```python
from build123d import *

# Parameters (mm, degrees)
SKETCH_1_W          = 56
SKETCH_1_H          = 104
SKETCH_1_R          = 1.6
EXTRUDE_1_DEPTH     = 2
FILLET_1_R          = 3
CUT_EXTRUDE_1_DEPTH = 10
FILLET_2_R          = 2


with BuildPart() as part:
    # 草图1 → 凸台-拉伸1 (new body)
    with BuildSketch(Plane.XY):
        Rectangle(SKETCH_1_W, SKETCH_1_H)
        with Locations((-24, 48)):
            Circle(SKETCH_1_R, mode=Mode.SUBTRACT)
        with Locations((-24, -48)):
            Circle(SKETCH_1_R, mode=Mode.SUBTRACT)
        with Locations(Location((24, -48, 0), (0, 0, 180))):
            Circle(SKETCH_1_R, mode=Mode.SUBTRACT)
        with Locations(Location((24, 48, 0), (0, 0, 180))):
            Circle(SKETCH_1_R, mode=Mode.SUBTRACT)
    extrude(amount=EXTRUDE_1_DEPTH)

    # 圆角1
    fillet_1_edges = [part.edges().sort_by_distance(p)[0] for p in [
        (28, -52, 1),
        (-28, -52, 1),
        (-28, 52, 1),
        (28, 52, 1),
    ]]
    fillet(fillet_1_edges, radius=FILLET_1_R)

    # 草图2 → 切除-拉伸1 (cut)
    with BuildSketch(Plane.XY.offset(2)):
        Polygon((-20, 34.939835194), (-20, -34.939835194), (-3.324169566, 0), align=None)
        Polygon((-17.198557706, -43), (17.198557706, -43), (0, -6.96492671), align=None)
        Polygon((0, 6.96492671), (-17.198557706, 43), (17.198557706, 43), align=None)
        Polygon((3.324169566, 0), (20, 34.939835194), (20, -34.939835194), align=None)
    extrude(amount=-CUT_EXTRUDE_1_DEPTH, mode=Mode.SUBTRACT)

    # 圆角2
    fillet_2_edges = [part.edges().sort_by_distance(p)[0] for p in [
        (-3.324169566, 0, 1),
        (-20, -34.939835194, 1),
        (-20, 34.939835194, 1),
        (-17.198557706, -43, 1),
        (0, -6.96492671, 1),
        (17.198557706, -43, 1),
        (17.198557706, 43, 1),
        (0, 6.96492671, 1),
        (-17.198557706, 43, 1),
        (20, -34.939835194, 1),
        (3.324169566, 0, 1),
        (20, 34.939835194, 1),
    ]]
    fillet(fillet_2_edges, radius=FILLET_2_R)


solid = part.part
```
Input: part model. Units: mm. Frame: model coordinates. A direction names the side the tool comes from. Round coordinates to 2 decimals unless told otherwise and drop trailing zeros. Loops run counter-clockwise (first coordinate to the right, second up) from the corner with the lowest first, then second, coordinate; pieces in that order, holes last. Notation, with made-up numbers: (-33.75, 86.5) -> (17.25, 86.5) arc R14 cw to (17.25, 106.5) -> close; hole circle Ø11 at (35.5, -10). An arc over 180 degrees is marked (long way). Use one line per item in the form item = value. Start each with the question number.
Item 1: Section query D-D on x = -5. Return the cut outline in (y, z), then the cut area to 3 significant figures.
Item 2: Material intervals for L1, parallel to Y at x = -24, z = 1.4; L2, parallel to Y at x = -11, z = 0.2; L3, parallel to X at y = -9.5, z = 1.75, sorted ascending. Write a range as from..to.
Item 3: Section query B-B on x = 24. Return the cut outline in (y, z).
Item 4: Set-up query: faces 4 (the face through (8.92, -25.65, 1.01)), 5 (the face through (0, -52, 1)). Return all of +Z, -Z, +X, -X, +Y, -Y with unobstructed straight access to the full face (end or side cutting, diameter ignored); none if empty.
Item 5: Section query C-C on y = -13.5. Return the cut outline in (x, z), then the cut area to 3 significant figures.
Item 6: Mould query, pull axis Y, two halves, no side actions, for faces 1 (the face through (-27.14, -51.1, 1.01)), 2 (the face through (0, 52, 1)), 3 (the face through (8.92, 25.65, 1.01)). Classes: pulls with the +Y half, pulls with the -Y half, needs draft (parallel to the pull), parting line crosses it, or undercut.
Item 7: Contact query for a flat-ended pin moving along its axis: pin 1 Ø1.9 at (x, y) = (-24, -48) entering from -Z. Output: stop coordinate, or through.
Item 8: Section query A-A on y = 48. Return the cut outline in (x, z), then the cut area to 3 significant figures.
Ans:
q1.outline = (-52, 0) -> (-43, 0) -> (-43, 2) -> (-52, 2) -> close; (-17.44, 0) -> (-3.51, 0) -> (-3.51, 2) -> (-17.44, 2) -> close; (3.51, 0) -> (17.44, 0) -> (17.44, 2) -> (3.51, 2) -> close; (43, 0) -> (52, 0) -> (52, 2) -> (43, 2) -> close
q1.area = 91.7 mm^2
q2.L1 = -52..-49.6, -46.4..46.4, 49.6..52
q2.L2 = -52..-43, -30.01..-16.08, 16.08..30.01, 43..52
q2.L3 = -28..-20, -7.86..7.86, 20..28
q3.outline = (-52, 0) -> (-49.6, 0) -> (-49.6, 2) -> (-52, 2) -> close; (-46.4, 0) -> (46.4, 0) -> (46.4, 2) -> (-46.4, 2) -> close; (49.6, 0) -> (52, 0) -> (52, 2) -> (49.6, 2) -> close
q4.face_4 = +Z, -Z
q4.face_5 = +Z, -Z, +X, -X, -Y
q5.outline = (-28, 0) -> (-20, 0) -> (-20, 2) -> (-28, 2) -> close; (-9.77, 0) -> (-3.12, 0) -> (-3.12, 2) -> (-9.77, 2) -> close; (3.12, 0) -> (9.77, 0) -> (9.77, 2) -> (3.12, 2) -> close; (20, 0) -> (28, 0) -> (28, 2) -> (20, 2) -> close
q5.area = 58.6 mm^2
q6.face_1 = pulls with the -Y half
q6.face_2 = pulls with the +Y half
q6.face_3 = undercut
q7.pin_1 = through
q8.outline = (-28, 0) -> (-25.6, 0) -> (-25.6, 2) -> (-28, 2) -> close; (-22.4, 0) -> (22.4, 0) -> (22.4, 2) -> (-22.4, 2) -> close; (25.6, 0) -> (28, 0) -> (28, 2) -> (25.6, 2) -> close
q8.area = 99.2 mm^2
